Design review of the part built by this model. Coordinates are the model's own, in mm. A direction names the side the tool comes from. Give positions to 0.01 mm unless a question says otherwise; leave off trailing zeros. Write each loop counter-clockwise with the first axis right and the second up, starting at its lowest first coordinate (ties: lowest second). Pieces come first, ordered by that corner, then holes.
```python
from build123d import *

# Parameters (mm, degrees)
CROQUIS1_W              = 40
CROQUIS1_H              = 76
CROQUIS1_R              = 3
SALIENTE_EXTRUIR1_DEPTH = 13
CROQUIS5_R              = 18.5
CORTAR_EXTRUIR3_DEPTH   = 6
CROQUIS6_R              = 1.5
CORTAR_EXTRUIR4_DEPTH   = 87.168439698
CROQUIS7_R              = 6
CORTAR_EXTRUIR5_DEPTH   = 6
CROQUIS8_R              = 2.35
CORTAR_EXTRUIR6_DEPTH   = 5
CORTAR_EXTRUIR7_START   = -5
CROQUIS9_R              = 2.35
CORTAR_EXTRUIR7_DEPTH   = 5


with BuildPart() as part:
    # Croquis1 → Saliente-Extruir1 (new body)
    with BuildSketch(Plane.XY):
        with Locations((20, 38)):
            Rectangle(CROQUIS1_W, CROQUIS1_H)
        with Locations(Location((20, 38, 0), (0, 0, 180))):
            Circle(CROQUIS1_R, mode=Mode.SUBTRACT)
    extrude(amount=SALIENTE_EXTRUIR1_DEPTH)

    # Croquis5 → Cortar-Extruir3 (cut)
    with BuildSketch(Plane(origin=(0, 0, 0), x_dir=(-1, 0, 0), z_dir=(0, 0, -1))):
        with Locations((-20, 45)):
            Circle(CROQUIS5_R)
    extrude(amount=-CORTAR_EXTRUIR3_DEPTH, mode=Mode.SUBTRACT)

    # Croquis6 → Cortar-Extruir4 (cut, through all)
    with BuildSketch(Plane(origin=(0, 0, 6), x_dir=(-1, 0, 0), z_dir=(0, 0, -1))):
        with Locations((-35.5, 45)):
            Circle(CROQUIS6_R)
        with Locations((-27.75, 58.423393759)):
            Circle(CROQUIS6_R)
        with Locations((-12.25, 58.423393759)):
            Circle(CROQUIS6_R)
        with Locations((-4.5, 45)):
            Circle(CROQUIS6_R)
        with Locations((-12.25, 31.576606241)):
            Circle(CROQUIS6_R)
        with Locations((-27.75, 31.576606241)):
            Circle(CROQUIS6_R)
    extrude(amount=-CORTAR_EXTRUIR4_DEPTH, mode=Mode.SUBTRACT)

    # Croquis7 → Cortar-Extruir5 (cut)
    with BuildSketch(Plane(origin=(0, 0, 6), x_dir=(-1, 0, 0), z_dir=(0, 0, -1))):
        with Locations((-20, 38)):
            Circle(CROQUIS7_R)
    extrude(amount=-CORTAR_EXTRUIR5_DEPTH, mode=Mode.SUBTRACT)

    # Croquis8 → Cortar-Extruir6 (cut)
    with BuildSketch(Plane(origin=(40, 0, 0), x_dir=(0, 0, -1), z_dir=(1, 0, 0))):
        with Locations((-6.5, 68)):
            Circle(CROQUIS8_R)
        with Locations((-6.5, 15)):
            Circle(CROQUIS8_R)
    extrude(amount=-CORTAR_EXTRUIR6_DEPTH, mode=Mode.SUBTRACT)

    # Croquis9 → Cortar-Extruir7 (cut)
    with BuildSketch(Plane.ZY.offset(CORTAR_EXTRUIR7_START)):
        with Locations(Location((6.5, 68, 0), (0, 0, 180))):
            Circle(CROQUIS9_R)
        with Locations(Location((6.5, 15, 0), (0, 0, 180))):
            Circle(CROQUIS9_R)
    extrude(amount=CORTAR_EXTRUIR7_DEPTH, mode=Mode.SUBTRACT)


solid = part.part
```
(1) Mouldability with a two-part tool opening along X and no side actions: class faces 1 (the face through (2.354, 50.557, 2.958)), 2 (the face through (22.21, 35.97, 12.49)), 3 (the face through (2.535, 17.085, 5.416)), 4 (the face through (40, 37, 6)) as pulls with the +X half, pulls with the -X half, needs draft (parallel to the pull), parting line crosses it, or undercut.
Resolved:
face 1: undercut
face 2: undercut
face 3: needs draft
face 4: pulls with the +X half
(2) Clearance check with flat-ended pins moving along their axes: P1, Ø1, axis at x = 24, y = 44, coming from the -Z side; P2, Ø2.5, axis at x = 12.25, y = 31.58, coming from the -Z side; P3, Ø2.5, axis at y = 15.5, z = 6.5, coming from the -X side; P4, Ø1.4, axis at y = 68, z = 7.5, coming from the +X side. State where each tip first meets the part, or that it passes through.
Resolved:
P1: stops at z = 6
P2: passes through
P3: stops at x = 5
P4: stops at x = 35
(3) To check wall thickness, follow L1, parallel to Y at x = 27.75, z = 8.25; L2, parallel to Y at x = 1.05, z = 6.5; L3, parallel to Y at x = 20, z = 3.7. State the ranges of each line that lie inside material, in increasing order.
Resolved:
L1: y = 0 to 30.08, 33.08 to 56.92, 59.92 to 76
L2: y = 0 to 12.65, 17.35 to 65.65, 70.35 to 76
L3: y = 0 to 26.5, 63.5 to 76
(4) Consider section B-B, the plane y = 45. Give the boundary of the cut face in (x, z), then the cut area to 3 significant figures.
Resolved:
outline: (0, 0) - (1.5, 0) - (1.5, 6) - (3, 6) - (3, 13) - (0, 13) - close; (6, 6) - (34, 6) - (34, 13) - (6, 13) - close; (37, 6) - (38.5, 6) - (38.5, 0) - (40, 0) - (40, 13) - (37, 13) - close
area: 256 mm2
(5) Tool access review of faces 5 (the face through (2.54, 65.67, 6.81)), 6 (the face through (24, 39, 13)), 7 (the face through (24.76, 34.35, 8.96)), 8 (the face through (20, 22, 0)), 9 (the face through (37.535, 12.915, 5.416)): name each direction out of +Z, -Z, +X, -X, +Y, -Y from which nothing blocks a thin tool from reaching the whole face with its end or side.
Resolved:
face 5: -X
face 6: +Z, +X, -X, +Y, -Y
face 7: -Z
face 8: -Z, +X, -X, +Y, -Y
face 9: +X
(6) Consider section C-C, the plane x = 28.5. Give the boundary of the cut face in (y, z), then the cut area to 3 significant figures.
Resolved:
outline: (0, 0) - (28.57, 0) - (28.57, 6) - (30.28, 6) - (30.28, 13) - (0, 13) - close; (32.88, 6) - (57.12, 6) - (57.12, 13) - (32.88, 13) - close; (59.72, 6) - (61.43, 6) - (61.43, 0) - (76, 0) - (76, 13) - (59.72, 13) - close
area: 754 mm2
(7) Consider section D-D, the plane y = 15. Give the boundary of the cut face in (x, z).
Resolved:
outline: (0, 0) - (40, 0) - (40, 4.15) - (35, 4.15) - (35, 8.85) - (40, 8.85) - (40, 13) - (0, 13) - (0, 8.85) - (5, 8.85) - (5, 4.15) - (0, 4.15) - close
(8) Consider section A-A, the plane x = 20. Give the boundary of the cut face in (y, z), then the cut area to 3 significant figures.
Resolved:
outline: (0, 0) - (26.5, 0) - (26.5, 6) - (32, 6) - (32, 12) - (35, 12) - (35, 13) - (0, 13) - close; (41, 12) - (44, 12) - (44, 6) - (63.5, 6) - (63.5, 0) - (76, 0) - (76, 13) - (41, 13) - close
area: 688 mm2
